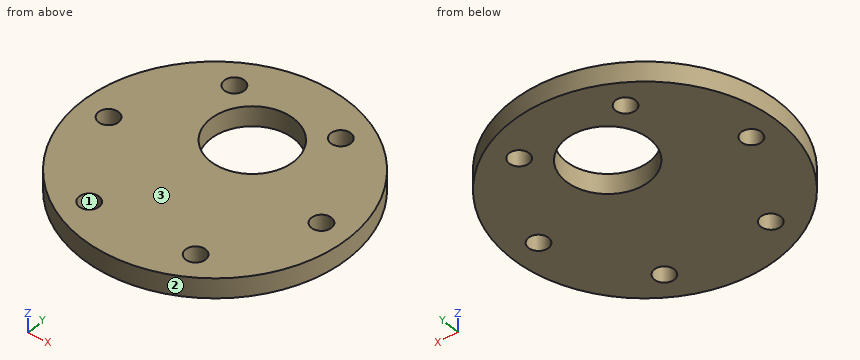
from build123d import *

# Parameters (mm, degrees)
SKETCH3_R               = 20
BOSS_EXTRUDE1_DEPTH     = 3
CUT_EXTRUDE2_DEPTH      = 29.442925307
CUT_EXTRUDE2_DEPTH_BACK = 29.442925307
SKETCH2_R               = 1.5
SKETCH2_R_2             = 6.25


with BuildPart() as part:
    # Sketch3 → Boss-Extrude1 (new body)
    with BuildSketch(Plane.XY):
        Circle(SKETCH3_R)
    extrude(amount=BOSS_EXTRUDE1_DEPTH)

    # Sketch2 → Cut-Extrude2 (cut, two sides: drawn at the far end of the back side and taken through both)
    with BuildSketch(Plane.XY.offset(-CUT_EXTRUDE2_DEPTH_BACK)):
        with Locations((-15.75, 0)):
            Circle(SKETCH2_R)
        with Locations((-7.875, 13.63990011)):
            Circle(SKETCH2_R)
        with Locations((7.875, 13.63990011)):
            Circle(SKETCH2_R)
        with Locations((15.75, 0)):
            Circle(SKETCH2_R)
        with Locations((7.875, -13.63990011)):
            Circle(SKETCH2_R)
        with Locations((-7.875, -13.63990011)):
            Circle(SKETCH2_R)
        with Locations((0, 7)):
            Circle(SKETCH2_R_2)
    extrude(amount=CUT_EXTRUDE2_DEPTH + CUT_EXTRUDE2_DEPTH_BACK, mode=Mode.SUBTRACT)


solid = part.part
Work out the finished part from the listing and answer in its coordinate system (mm). Face numbers are marked on the shaded views. Give positions to 0.01 mm unless a question says otherwise; leave off trailing zeros. Loops run counter-clockwise (first coordinate to the right, second up) from the corner with the lowest first, then second, coordinate; pieces in that order, holes last. Notation, with made-up numbers: (65, 42.25) -> (72, 42.25) arc R13 cw to (72, 62.25) -> close; hole circle Ø9 at (-19.5, -11.75). An arc over 180 degrees is marked (long way). Use a Markdown table: item, result. Add a question column.
1. Section D-D on x = 8.5 is taken. Determine the outline of the cut face in (y, z), and give its area (3 significant figures).
2. Flat-ended cylindrical pins translate along their axes: pin 1 Ø1 at (x, z) = (11, 1.5) entering from +Y; pin 2 Ø1 at (y, z) = (-12, 2.5) entering from +X. Find the tip coordinate at first contact, or state that the pin passes through.
3. Find the intervals of material crossed by probe 1 along Y at (x, z) = (15.75, 1.55); probe 2 along X at (y, z) = (11.5, 1.2); probe 3 along Y at (x, z) = (3, 1.4), in increasing order.
4. Section A-A on x = 0 is taken. Determine the outline of the cut face in (y, z).
5. Section C-C on y = 10 is taken. Determine the outline of the cut face in (x, z).
6. Section B-B on z = 1.6 is taken. Determine the outline of the cut face in (x, y) (3 decimals), and give its area (3 significant figures).
7. Determine the mould class of the marked faces 1, 2 and 3 for opening direction Y: released by +Y, released by -Y, zero draft, split by the parting line, or undercut.
Results below:
| question | item | result |
|---|---|---|
| 1 | outline | (-18.1, 0) -> (-15, 0) -> (-15, 3) -> (-18.1, 3) -> close; (-12.28, 0) -> (12.28, 0) -> (12.28, 3) -> (-12.28, 3) -> close; (15, 0) -> (18.1, 0) -> (18.1, 3) -> (15, 3) -> close |
| 1 | area | 92.3 mm^2 |
| 2 | pin 1 | stops at y = 17.02 |
| 2 | pin 2 | stops at x = 16.36 |
| 3 | probe 1 | y = -12.33 to -1.5, 1.5 to 12.33 |
| 3 | probe 2 | x = -16.36 to -4.34, 4.34 to 16.36 |
| 3 | probe 3 | y = -19.77 to 1.52, 12.48 to 19.77 |
| 4 | outline | (-20, 0) -> (0.75, 0) -> (0.75, 3) -> (-20, 3) -> close; (13.25, 0) -> (20, 0) -> (20, 3) -> (13.25, 3) -> close |
| 5 | outline | (-17.32, 0) -> (-5.48, 0) -> (-5.48, 3) -> (-17.32, 3) -> close; (5.48, 0) -> (17.32, 0) -> (17.32, 3) -> (5.48, 3) -> close |
| 6 | outline | circle Ø40 at (0, 0); hole circle Ø3 at (-15.75, 0); hole circle Ø3 at (-7.875, -13.64); hole circle Ø3 at (-7.875, 13.64); hole circle Ø12.5 at (0, 7); hole circle Ø3 at (7.875, -13.64); hole circle Ø3 at (7.875, 13.64); hole circle Ø3 at (15.75, 0) |
| 6 | area | 1,090 mm^2 |
| 7 | face 1 | undercut |
| 7 | face 2 | split by the parting line |
| 7 | face 3 | zero draft |
